from build123d import *

# Parameters (mm, degrees)
F0_W      = 127
F0_H      = 127
F1_DEPTH  = 127
F2_R      = 12.7
F3_DEPTH  = 6.35
F4_R      = 12.7
F5_DEPTH  = 6.35
F6_R      = 12.7
F7_R      = 12.7
F7_R_2    = 12.14507
F8_DEPTH  = 6.35
F9_R      = 12.7
F10_DEPTH = 6.35
F11_R     = 12.7
F12_DEPTH = 6.35
F13_R     = 12.7
F14_DEPTH = 6.35


with BuildPart() as f1:
    # F0 (on Top) → F1 (new body)
    with BuildSketch(Plane.XY):
        with Locations((63.5, -63.5)):
            Rectangle(F0_W, F0_H)
    extrude(amount=F1_DEPTH)

    # F2 (on face) → F3 (cut)
    with BuildSketch(Plane.YZ.offset(127)):
        with Locations((-63.5, 63.5)):
            Circle(F2_R)
    extrude(amount=-F3_DEPTH, mode=Mode.SUBTRACT)

    # F4 (on face) → F5 (cut)
    with BuildSketch(Plane.XZ.offset(127)):
        with Locations((20.24712, 105.882019)):
            Circle(F4_R)
        with Locations((104.775, 22.225)):
            Circle(F4_R)
    extrude(amount=-F5_DEPTH, mode=Mode.SUBTRACT)

    # F6 (on face) + F7 (on face) → F8 (cut)
    with BuildSketch(Plane(origin=(0, 0, 0), x_dir=(0, -1, 0), z_dir=(-1, 0, 0))):
        with Locations((107.403494, 21.579256)):
            Circle(F6_R)
    with BuildSketch(Plane(origin=(0, 0, 0), x_dir=(0, -1, 0), z_dir=(-1, 0, 0))):
        with Locations((63.5, 22.225)):
            Circle(F7_R)
        with Locations((22.247186, 24.020914)):
            Circle(F7_R_2)
        with Locations((104.775, 104.775)):
            Circle(F7_R)
        with Locations((63.5, 104.775)):
            Circle(F7_R)
        with Locations((22.225, 104.775)):
            Circle(F7_R_2)
    extrude(amount=-F8_DEPTH, mode=Mode.SUBTRACT)

    # F9 (on face) → F10 (cut)
    with BuildSketch(Plane(origin=(0, 0, 0), x_dir=(-1, 0, 0), z_dir=(0, 1, 0))):
        with Locations((-22.44245, 104.347)):
            Circle(F9_R)
        with Locations((-63.5, 63.5)):
            Circle(F9_R)
        with Locations((-22.44245, 22.653)):
            Circle(F9_R)
        with Locations((-104.775, 22.225)):
            Circle(F9_R)
        with Locations((-104.775, 104.775)):
            Circle(F9_R)
    extrude(amount=-F10_DEPTH, mode=Mode.SUBTRACT)

    # F11 (on face) → F12 (cut)
    with BuildSketch(Plane(origin=(0, 0, 0), x_dir=(1, 0, 0), z_dir=(0, 0, -1))):
        with Locations((104.775, 104.775)):
            Circle(F11_R)
        with Locations((22.225, 104.775)):
            Circle(F11_R)
        with Locations((104.775, 22.225)):
            Circle(F11_R)
        with Locations((22.225, 22.225)):
            Circle(F11_R)
    extrude(amount=-F12_DEPTH, mode=Mode.SUBTRACT)

    # F13 (on face) → F14 (cut)
    with BuildSketch(Plane.XY.offset(127)):
        with Locations((63.5, -63.5)):
            Circle(F13_R)
        with Locations((104.775, -104.775)):
            Circle(F13_R)
        with Locations((22.225, -22.225)):
            Circle(F13_R)
    extrude(amount=-F14_DEPTH, mode=Mode.SUBTRACT)


solid = f1.part
Work out the finished part from the listing and answer in its coordinate system (mm). A direction names the side the tool comes from. Round coordinates to 2 decimals unless told otherwise and drop trailing zeros. Write each loop counter-clockwise with the first axis right and the second up, starting at its lowest first coordinate (ties: lowest second). Pieces come first, ordered by that corner, then holes. Notation, with made-up numbers: M -35,77 L 13,77 A20 ccw 13,83 Z; hole C -16.75,44.5 d2. An arc over 180 degrees is marked long. Use a Markdown table: item, result.
1) The part is cut by section C-C on z = 63.5. Give the vertices of the cut face in (x, y), plus the area to 3 significant figures.
Taken from the geometry:
| item | result |
|---|---|
| outline | M 0,-127 L 127,-127 L 127,-76.2 L 120.65,-76.2 L 120.65,-50.8 L 127,-50.8 L 127,0 L 76.2,0 L 76.2,-6.35 L 50.8,-6.35 L 50.8,0 L 0,0 Z |
| area | 15,800 mm2 |
2) Which of the six approach directions +Z, -Z, +X, -X, +Y, -Y give full straight-line access (tool end or side, diameter ignored) to faces 4 (the face through (18.594, -123.869, 118.474)), 5 (the face through (6.35, -105, 105)), 6 (the face through (75.614, -59.685, 123.869))?
Taken from the geometry:
| item | result |
|---|---|
| face 4 | -Y |
| face 5 | -X |
| face 6 | +Z |
3) The part is cut by section B-B on x = 63.5. Give the vertices of the cut face in (y, z).
Taken from the geometry:
| item | result |
|---|---|
| outline | M -127,0 L 0,0 L 0,50.8 L -6.35,50.8 L -6.35,76.2 L 0,76.2 L 0,127 L -50.8,127 L -50.8,120.65 L -76.2,120.65 L -76.2,127 L -127,127 Z |
4) Flat-ended cylindrical pins translate along their axes: pin 1 (15 mm diameter, centred on x = 22.225, y = -22.225, fed in from +Z); pin 2 (15 mm diameter, centred on x = 20.25, z = 105.88, fed in from +Y); pin 3 (12 mm diameter, centred on y = -16.5, z = 25, fed in from -X). Find the tip coordinate at first contact, or state that the pin passes through.
Taken from the geometry:
| item | result |
|---|---|
| pin 1 | stops at z = 120.65 |
| pin 2 | stops at y = -6.35 |
| pin 3 | stops at x = 6.35 |
5) Determine the mould class of faces 1 (the face through (19.472, -9.827, 3.131)), 2 (the face through (6.35, -63, 22)), 3 (the face through (3.13, -28.75, 115.02)) for opening direction X: pulls with the +X half, pulls with the -X half, needs draft (parallel to the pull), parting line crosses it, or undercut.
Taken from the geometry:
| item | result |
|---|---|
| face 1 | undercut |
| face 2 | pulls with the -X half |
| face 3 | needs draft |
6) The part is cut by section A-A on y = -63.5. Give the vertices of the cut face in (x, z) (3 decimals).
Taken from the geometry:
| item | result |
|---|---|
| outline | M 0,0 L 127,0 L 127,50.8 L 120.65,50.8 L 120.65,76.2 L 127,76.2 L 127,127 L 76.2,127 L 76.2,120.65 L 50.8,120.65 L 50.8,127 L 0,127 L 0,117.475 L 6.35,117.475 L 6.35,92.075 L 0,92.075 L 0,34.925 L 6.35,34.925 L 6.35,9.525 L 0,9.525 Z |
7) Consider line 1 (Z direction, x = 63, y = -3); line 2 (Y direction, x = 63.5, z = 122.75). Determine where each line is inside the solid, lowest interval first. Write a range as [from, to].
Taken from the geometry:
| item | result |
|---|---|
| line 1 | z = [0, 50.81], [76.19, 127] |
| line 2 | y = [-127, -76.2], [-50.8, 0] |
8) The part is cut by section D-D on z = 32. Give the vertices of the cut face in (x, y), plus the area to 3 significant figures.
Taken from the geometry:
| item | result |
|---|---|
| outline | M 0,-127 L 96.67,-127 L 96.67,-120.65 L 112.88,-120.65 L 112.88,-127 L 127,-127 L 127,0 L 112.88,0 L 112.88,-6.35 L 96.67,-6.35 L 96.67,0 L 31.04,0 L 31.04,-6.35 L 13.84,-6.35 L 13.84,0 L 0,0 L 0,-13.09 L 6.35,-13.09 L 6.35,-31.4 L 0,-31.4 L 0,-55.39 L 6.35,-55.39 L 6.35,-71.61 L 0,-71.61 L 0,-100.14 L 6.35,-100.14 L 6.35,-114.66 L 0,-114.66 Z |
| area | 15,500 mm2 |
